Check sheet for the modelled part. Datum: model origin and axes. Units: mm. A direction names the side the tool comes from. Coordinates: 2 decimals unless noted, no trailing zeros. Write each loop counter-clockwise with the first axis right and the second up, starting at its lowest first coordinate (ties: lowest second). Pieces come first, ordered by that corner, then holes. Notation, with made-up numbers: M 37,31.25 L 64,31.25 A27 ccw 64,48.25 Z; hole C -29.5,16.5 d1. An arc over 180 degrees is marked long. Answer as CSV lines item,"result". Start each with the question number.
Q1. Sectioned sample at A-A, the plane y = -72.95. Record the cut outline in (x, z).
Q2. Thickness scan on line 1 along Z through (x, y) = (75.5, -72.9); line 2 along X through (y, z) = (-74.1, -1.5). Record the ranges inside material, lowest first. Write a range as from..to.
Q3. Access from +Z, -Z, +X, -X, +Y, -Y to the whole of each face (thin tool, end or side, straight path). Record for faces 1 (the flat face through (73, -74, 0)), 2 (the flat face through (115, -72.5, 15)), 3 (the flat face through (148, -74, 34)), 4 (the flat face through (155, -74, 0)), 5 (the flat face through (78, -74, 34)).
Q4. Depth check by flat-ended pin: pin 1 Ø0.6 at (y, z) = (-73, 34) entering from -X; pin 2 Ø1 at (x, y) = (155.5, -73.5) entering from -Z; pin 3 Ø0.6 at (x, y) = (73, -73.5) entering from +Z. Enter the tip coordinate at first touch or a pass-through.
from build123d import *

# Parameters (mm, degrees)
ESTRUSIONE_ESTRUSIONE1_DEPTH      = 35.42788
ESTRUSIONE_ESTRUSIONE1_DEPTH_BACK = 4.57212
SCHIZZO1_W                        = 70
SCHIZZO1_H                        = 2
SCHIZZO2_W                        = 33.42788034
SCHIZZO2_H                        = 2
ESTRUSIONE_ESTRUSIONE2_DEPTH      = 15
SCHIZZO3_W                        = 33.42788034
SCHIZZO3_H                        = 2
ESTRUSIONE_ESTRUSIONE3_DEPTH      = 10


with BuildPart() as part:
    # Schizzo1 → Estrusione-Estrusione1 (new, two sides: drawn at the far end of the back side and taken through both)
    with BuildSketch(Plane.XY.offset(-ESTRUSIONE_ESTRUSIONE1_DEPTH_BACK)):
        with Locations((113, -73.5)):
            Rectangle(SCHIZZO1_W, SCHIZZO1_H)
    extrude(amount=ESTRUSIONE_ESTRUSIONE1_DEPTH + ESTRUSIONE_ESTRUSIONE1_DEPTH_BACK)

    # Schizzo2 → Estrusione-Estrusione2 (add)
    with BuildSketch(Plane(origin=(148, 0, 0), x_dir=(0, 0, -1), z_dir=(1, 0, 0))):
        with Locations((-16.71394017, -73.5)):
            Rectangle(SCHIZZO2_W, SCHIZZO2_H)
    extrude(amount=ESTRUSIONE_ESTRUSIONE2_DEPTH)

    # Schizzo3 → Estrusione-Estrusione3 (add)
    with BuildSketch(Plane.ZY.offset(-78)):
        with Locations((16.71394017, -73.5)):
            Rectangle(SCHIZZO3_W, SCHIZZO3_H)
    extrude(amount=ESTRUSIONE_ESTRUSIONE3_DEPTH)


solid = part.part
Output:
1,outline,"M 68,0 L 78,0 L 78,-4.57 L 148,-4.57 L 148,0 L 163,0 L 163,33.43 L 148,33.43 L 148,35.43 L 78,35.43 L 78,33.43 L 68,33.43 Z"
2,line 1,"z = 0..33.43"
2,line 2,"x = 78..148"
3,face 1,"-Z, -X, +Y, -Y"
3,face 2,"+Z, -Z, +X, -X, +Y"
3,face 3,"+Z, +X, +Y, -Y"
3,face 4,"-Z, +X, +Y, -Y"
3,face 5,"+Z, -X, +Y, -Y"
4,pin 1,"stops at x = 78"
4,pin 2,"stops at z = 0"
4,pin 3,"stops at z = 33.43"
